Part model, mm, in its own coordinate system. Face numbers are marked on the shaded views. A direction names the side the tool comes from. Coordinates: 2 decimals unless noted, no trailing zeros. Loops run counter-clockwise (first coordinate to the right, second up) from the corner with the lowest first, then second, coordinate; pieces in that order, holes last. Notation, with made-up numbers: M 66.5,29 L 106.5,29 A34 cw 106.5,63 Z; hole C 30.25,73 d4. An arc over 180 degrees is marked long. Answer as a JSON object with one key per item and string values. Group by question number.
1. Saw through at D-D on x = -2. Write the cut outline in (y, z), then the cut area to 3 significant figures.
2. Drop flat-ended pins along their axis: pin 1 Ø1 at (y, z) = (2, 7) entering from +X; pin 2 Ø1.6 at (x, z) = (-1.5, -1.5) entering from +Y; pin 3 Ø1.1 at (x, z) = (2, 0.5) entering from -Y. Give the stop position or say it passes through.
3. Saw through at A-A on z = -2. Write the cut outline in (x, y), then the cut area to 3 significant figures.
4. Saw through at B-B on x = -1.15. Write the cut outline in (y, z).
5. Mould opens along Z. For the marked faces 4, 5 and 6 say: released by +Z, released by -Z, zero draft, split by the parting line, or undercut.
6. Saw through at C-C on y = -0.75. Write the cut outline in (x, z).
7. 3-axis set-ups, long thin cutter, end or side, ignore diameter. For the marked faces 1, 2 and 3: which of +Z, -Z, +X, -X, +Y, -Y reach the whole face in a straight line?
8. Drill centre lines: L1, parallel to Z at x = 1.9, y = 1.55; L2, parallel to X at y = 0, z = -4.5; L3, parallel to Z at x = -1.8, y = -0.45. Where is each one in solid material? Low to high.
from build123d import *

# Parameters (mm, degrees)
F0_R      = 2.35
F0_R_2    = 1.6
F1_DEPTH  = 7.9
F3_DEPTH  = 3
F0_R_3    = 2.9
F4_DEPTH  = 0.9
F5_W      = 1.8
F5_H      = 7
F6_DEPTH  = 12.5
F7_R      = 0.5
F9_DEPTH  = 3
F10_R     = 0.3999
F12_DEPTH = 0.3
F14_DEPTH = 0.3
F16_DEPTH = 0.3


# Not quite as in the source:
# - a fillet or chamfer is up to 0.001 mm smaller than in the source, because OpenCascade refuses the exact size


with BuildPart() as f1:
    # F0 (on Top) → F1 (new body, symmetric)
    with BuildSketch(Plane.XY):
        Circle(F0_R)
        Circle(F0_R_2, mode=Mode.SUBTRACT)
    extrude(amount=F1_DEPTH, both=True)

    # F2 (on face) → F3 (cut)
    with BuildSketch(Plane.XY.offset(7.9)):
        with BuildLine():
            ThreePointArc((-0.4, 1.5491933385), (-0.201606868, 1.587247514), (0, 1.6))
            ThreePointArc((0, 1.6), (0.201606868, 1.587247514), (0.4, 1.5491933385))
            Line((0.4, 1.5491933385), (0.4, 1.6))
            Line((0.4, 1.6), (0.4, 2.3157072354))
            ThreePointArc((0.4, 2.3157072354), (0, 2.35), (-0.4, 2.3157072354))
            Line((-0.4, 2.3157072354), (-0.4, 1.6))
            Line((-0.4, 1.6), (-0.4, 1.5491933385))
        make_face()
        with BuildLine():
            ThreePointArc((0.4, -1.5491933385), (0.201606868, -1.587247514), (0, -1.6))
            ThreePointArc((0, -1.6), (-0.201606868, -1.587247514), (-0.4, -1.5491933385))
            Line((-0.4, -1.5491933385), (-0.4, -1.6))
            Line((-0.4, -1.6), (-0.4, -2.3157072354))
            ThreePointArc((-0.4, -2.3157072354), (0, -2.35), (0.4, -2.3157072354))
            Line((0.4, -2.3157072354), (0.4, -1.6))
            Line((0.4, -1.6), (0.4, -1.5491933385))
        make_face()
    extrude(amount=-F3_DEPTH, mode=Mode.SUBTRACT)

    # F0 (on Top) → F4 (join, symmetric)
    with BuildSketch(Plane.XY):
        Circle(F0_R_3)
        Circle(F0_R, mode=Mode.SUBTRACT)
    extrude(amount=F4_DEPTH, both=True)

    # F5 (on Right) → F6 (cut, symmetric)
    with BuildSketch(Plane.YZ):
        Rectangle(F5_W, F5_H)
    extrude(amount=F6_DEPTH, both=True, mode=Mode.SUBTRACT)

    # F7
    f7_edges = [f1.edges().sort_by_distance(p)[0] for p in [
        (-1.746852, -0.9, 3.5),
        (1.746852, -0.9, 3.5),
        (1.746852, 0.9, 3.5),
        (-1.746852, 0.9, 3.5),
        (1.746852, -0.9, -3.5),
        (-1.746852, -0.9, -3.5),
        (1.746852, 0.9, -3.5),
        (-1.746852, 0.9, -3.5),
    ]]
    fillet(f7_edges, radius=F7_R)

    # F8 (on face) → F9 (cut)
    with BuildSketch(Plane(origin=(0, 0, -7.9), x_dir=(1, 0, 0), z_dir=(0, 0, -1))):
        with BuildLine():
            Line((0.4, 1.5491933385), (0.4, 1.6))
            Line((0.4, 1.6), (0.4, 2.3157072354))
            ThreePointArc((0.4, 2.3157072354), (0, 2.35), (-0.4, 2.3157072354))
            Line((-0.4, 2.3157072354), (-0.4, 1.6))
            Line((-0.4, 1.6), (-0.4, 1.5491933385))
            ThreePointArc((-0.4, 1.5491933385), (0, 1.6), (0.4, 1.5491933385))
        make_face()
        with BuildLine():
            ThreePointArc((-0.4, -2.3157072354), (0, -2.35), (0.4, -2.3157072354))
            Line((0.4, -2.3157072354), (0.4, -1.6))
            Line((0.4, -1.6), (0.4, -1.5491933385))
            ThreePointArc((0.4, -1.5491933385), (0, -1.6), (-0.4, -1.5491933385))
            Line((-0.4, -1.5491933385), (-0.4, -1.6))
            Line((-0.4, -1.6), (-0.4, -2.3157072354))
        make_face()
    extrude(amount=-F9_DEPTH, mode=Mode.SUBTRACT)

    # F10 (radius 0.4 in the source; OpenCascade refuses exactly that, so slightly less here)
    f10_edges = [f1.edges().sort_by_distance(p)[0] for p in [
        (0.4, -1.93245, -4.9),
        (-0.4, -1.93245, -4.9),
        (-0.4, 1.93245, -4.9),
        (0.4, 1.93245, -4.9),
        (0.4, 1.93245, 4.9),
        (-0.4, 1.93245, 4.9),
        (-0.4, -1.93245, 4.9),
        (0.4, -1.93245, 4.9),
    ]]
    fillet(f10_edges, radius=F10_R)

    # F11 (on face) → F12 (join)
    with BuildSketch(Plane(origin=(0, 0, -7.9), x_dir=(1, 0, 0), z_dir=(0, 0, -1))):
        with BuildLine():
            Line((-0.4, 2.3157072354), (-0.4, 2.4677925359))
            ThreePointArc((-0.4, 2.4677925359), (-2.5, 0), (-0.4, -2.4677925359))
            Line((-0.4, -2.4677925359), (-0.4, -2.3157072354))
            ThreePointArc((-0.4, -2.3157072354), (-2.35, 0), (-0.4, 2.3157072354))
        make_face()
        with BuildLine():
            ThreePointArc((0.4, -2.4677925359), (1.9039432765, -1.6201851746), (2.5, 0))
            ThreePointArc((2.5, 0), (1.9039432765, 1.6201851746), (0.4, 2.4677925359))
            Line((0.4, 2.4677925359), (0.4, 2.3157072354))
            ThreePointArc((0.4, 2.3157072354), (1.7975678012, 1.5136875503), (2.35, 0))
            ThreePointArc((2.35, 0), (1.7975678012, -1.5136875503), (0.4, -2.3157072354))
            Line((0.4, -2.3157072354), (0.4, -2.4677925359))
        make_face()
    extrude(amount=-F12_DEPTH)

    # F13 (on face) → F14 (join)
    with BuildSketch(Plane.XY.offset(7.9)):
        with BuildLine():
            Line((-0.4, 2.3157072354), (-0.4, 2.4677925359))
            ThreePointArc((-0.4, 2.4677925359), (-2.5, 0), (-0.4, -2.4677925359))
            Line((-0.4, -2.4677925359), (-0.4, -2.3157072354))
            ThreePointArc((-0.4, -2.3157072354), (-2.35, 0), (-0.4, 2.3157072354))
        make_face()
    extrude(amount=-F14_DEPTH)

    # F15 (on face) → F16 (join)
    with BuildSketch(Plane.XY.offset(7.9)):
        with BuildLine():
            ThreePointArc((0.4, -2.4677925359), (1.9039432765, -1.6201851746), (2.5, 0))
            ThreePointArc((2.5, 0), (1.9039432765, 1.6201851746), (0.4, 2.4677925359))
            Line((0.4, 2.4677925359), (0.4, 2.3157072354))
            ThreePointArc((0.4, 2.3157072354), (1.7975678012, 1.5136875503), (2.35, 0))
            ThreePointArc((2.35, 0), (1.7975678012, -1.5136875503), (0.4, -2.3157072354))
            Line((0.4, -2.3157072354), (0.4, -2.4677925359))
        make_face()
    extrude(amount=-F16_DEPTH)


solid = f1.part
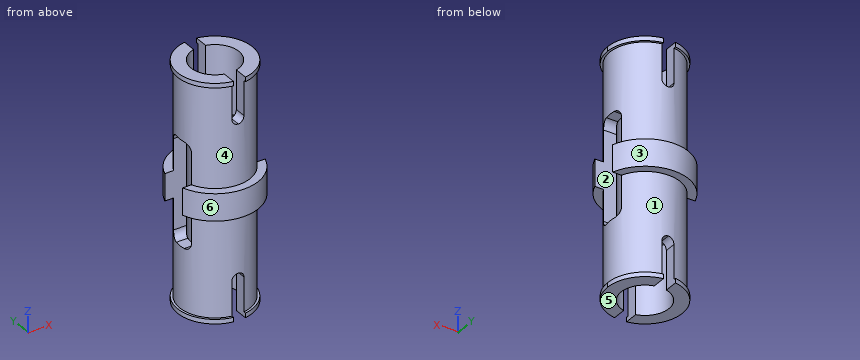
Outcome:
{
 "1": {"outline": "M -2.1,-0.9 L -1.23,-0.9 L -1.23,-7.6 L -1.5,-7.6 L -1.5,-7.9 L 1.5,-7.9 L 1.5,-7.6 L 1.23,-7.6 L 1.23,-0.9 L 2.1,-0.9 L 2.1,0.9 L 1.23,0.9 L 1.23,7.6 L 1.5,7.6 L 1.5,7.9 L -1.5,7.9 L -1.5,7.6 L -1.23,7.6 L -1.23,0.9 L -2.1,0.9 Z; hole M -0.9,-3 A0.5 ccw -0.4,-3.5 L 0.4,-3.5 A0.5 ccw 0.9,-3 L 0.9,3 A0.5 ccw 0.4,3.5 L -0.4,3.5 A0.5 ccw -0.9,3 Z", "area": "30.0 mm²"},
 "2": {"pin 1": "stops at x = 1.81", "pin 2": "stops at y = 2.73", "pin 3": "stops at y = -2.51"},
 "3": {"outline": "M -2.17,-0.9 A2.35 ccw 2.17,-0.9 L 1.32,-0.9 A1.6 cw -1.32,-0.9 Z; M -2.17,0.9 L -1.32,0.9 A1.6 cw 1.32,0.9 L 2.17,0.9 A2.35 ccw Z", "area": "6.50 mm²"},
 "4": {"outline": "M -2.66,-0.9 L -2.05,-0.9 L -2.05,-7.6 L -2.22,-7.6 L -2.22,-7.9 L -1.11,-7.9 L -1.11,7.9 L -2.22,7.9 L -2.22,7.6 L -2.05,7.6 L -2.05,0.9 L -2.66,0.9 Z; M 1.11,-7.9 L 2.22,-7.9 L 2.22,-7.6 L 2.05,-7.6 L 2.05,-0.9 L 2.66,-0.9 L 2.66,0.9 L 2.05,0.9 L 2.05,7.6 L 2.22,7.6 L 2.22,7.9 L 1.11,7.9 Z"},
 "5": {"face 4": "undercut", "face 5": "released by -Z", "face 6": "zero draft"},
 "6": {"outline": "M -2.38,-7.9 L -1.41,-7.9 L -1.41,-3.36 L -2.23,-3.36 L -2.23,-7.6 L -2.38,-7.6 Z; M -2.38,7.6 L -2.23,7.6 L -2.23,3.36 L -1.41,3.36 L -1.41,7.9 L -2.38,7.9 Z; M 1.41,-7.9 L 2.38,-7.9 L 2.38,-7.6 L 2.23,-7.6 L 2.23,-3.36 L 1.41,-3.36 Z; M 1.41,3.36 L 2.23,3.36 L 2.23,7.6 L 2.38,7.6 L 2.38,7.9 L 1.41,7.9 Z"},
 "7": {"face 1": "none", "face 2": "+X, -X", "face 3": "+Z, -Z, +Y"},
 "8": {"L1": "z = -7.9 to -7.6, -0.9 to 0.9, 7.6 to 7.9", "L2": "x = -2.35 to -1.6, 1.6 to 2.35", "L3": "z = -7.9 to -3.5, 3.5 to 7.9"}
}
